The model under review builds one solid part; all positions refer to its coordinate system, in mm. A direction names the side the tool comes from. Give positions to 0.01 mm unless a question says otherwise; leave off trailing zeros. Order: outer loops, then holes, each group sorted by start corner. A loop starts at its lowest first (then second) coordinate and runs counter-clockwise, first axis right, second up. Notation, with made-up numbers: (27.5, 18) - (76.5, 18) arc R20 ccw to (76.5, 52) - close; hole circle Ø3 at (-33, 59.25). An arc over 180 degrees is marked (long way). Put each result on its own line as item: value.
```python
from build123d import *

# Parameters (mm, degrees)
F0_W     = 100.278783
F0_H     = 100.845326
F1_DEPTH = 10
F3_DEPTH = 2
F4_W     = 20.395683
F4_H     = 3.682554
F5_DEPTH = 2
F7_DEPTH = 2


with BuildPart() as f1:
    # F0 (on Top) → F1 (new body)
    with BuildSketch(Plane.XY):
        with Locations((14.022036, -22.520235)):
            Rectangle(F0_W, F0_H)
    extrude(amount=F1_DEPTH)

    # F2 (on face) → F3 (join)
    with BuildSketch(Plane.XY.offset(10)):
        Polygon((7.790018, 0), (0, 0), (0, -27.335884), (-3.824191, -31.301711), (-3.824191, -49.71448), (6.940198, -60.478866), (32.718081, -60.478866), (38.950093, -50.847575), (38.950093, -31.584986), (33.567898, -27.335884), (33.567898, 0), (25.352968, 0), (25.352968, -13.738759), (7.790018, -13.738759), align=None)
    extrude(amount=F3_DEPTH)

    # F4 (on face) → F5 (join)
    with BuildSketch(Plane.XY.offset(12)):
        with Locations((17.987859, -37.675362)):
            Rectangle(F4_W, F4_H)
    extrude(amount=-F5_DEPTH)

    # F6 (on face) → F7 (join)
    with BuildSketch(Plane.XY.offset(12)):
        Polygon((28.752247, -32.718077), (5.523832, -33.567894), (5.523832, -38.666818), (28.752247, -38.666818), align=None)
    extrude(amount=F7_DEPTH)


solid = f1.part
```
(1) Wall thickness on L1, parallel to Z at x = -10, y = -66; L2, parallel to Y at x = 20.5, z = 12.25: over which ranges is each line inside the solid? List them lowest first.
The answers:
L1: 0 to 10
L2: -38.67 to -33.02
(2) Take a section at B-B, the plane x = 36.5. Write out the cut boundary in (y, z).
The answers:
outline: (-72.94, 0) - (27.9, 0) - (27.9, 10) - (-29.65, 10) - (-29.65, 12) - (-54.63, 12) - (-54.63, 10) - (-72.94, 10) - close
(3) Clearance check with flat-ended pins moving along their axes: pin 1 Ø0.6 at (y, z) = (-13.5, 11.5) entering from -X; pin 2 Ø1 at (y, z) = (-10, 11) entering from +X; pin 3 Ø3 at (x, z) = (-22.5, 12) entering from +Y; pin 4 Ø1.6 at (x, z) = (20, 11.5) entering from +Y. State where each tip first meets the part, or that it passes through.
The answers:
pin 1: x = 0
pin 2: x = 33.57
pin 3: through
pin 4: y = -13.74
(4) Take a section at D-D, the plane x = 24. Write out the cut boundary in (y, z), then the cut area to 3 significant figures.
The answers:
outline: (-72.94, 0) - (27.9, 0) - (27.9, 10) - (-13.74, 10) - (-13.74, 12) - (-32.89, 12) - (-32.89, 14) - (-38.67, 14) - (-38.67, 12) - (-60.48, 12) - (-60.48, 10) - (-72.94, 10) - close
area: 1,110 mm^2
(5) Take a section at A-A, the plane y = -35.5. Write out the cut boundary in (x, z).
The answers:
outline: (-36.12, 0) - (64.16, 0) - (64.16, 10) - (38.95, 10) - (38.95, 12) - (28.75, 12) - (28.75, 14) - (5.52, 14) - (5.52, 12) - (-3.82, 12) - (-3.82, 10) - (-36.12, 10) - close
(6) For faces 1 (the flat face through (-1.885, -29.291, 10.986)), 2 (the flat face through (35.79, -55.73, 10.99)), 3 (the flat face through (36.297, -29.49, 10.986)), list the 3-axis set-ups (+Z, -Z, +X, -X, +Y, -Y) from which the entire face can be reached by the end or side of a thin tool; tool diameter is ignored.
The answers:
face 1: +Z, -X, +Y
face 2: +Z, +X, -Y
face 3: +Z, +X, +Y
(7) Take a section at C-C, the plane y = -47. Write out the cut boundary in (x, z).
The answers:
outline: (-36.12, 0) - (64.16, 0) - (64.16, 10) - (38.95, 10) - (38.95, 12) - (-3.82, 12) - (-3.82, 10) - (-36.12, 10) - close
